Could you check a few things on this model? Use its own coordinates, in mm. A direction names the side the tool comes from. Round coordinates to 2 decimals unless told otherwise and drop trailing zeros. Loops run counter-clockwise (first coordinate to the right, second up) from the corner with the lowest first, then second, coordinate; pieces in that order, holes last.
from build123d import *

# Parameters (mm, degrees)
SKETCH1_W           = 109.51405142
SKETCH1_H           = 53
SKETCH1_R           = 1.75
BOSS_EXTRUDE1_DEPTH = 30
SKETCH2_W           = 93.51405142
SKETCH2_H           = 27.46
CUT_EXTRUDE1_DEPTH  = 239.893281613
SKETCH4_W           = 53.34
SKETCH4_H           = 27.94
CUT_EXTRUDE3_DEPTH  = 239.587618287
SKETCH5_W           = 56.34
SKETCH5_H           = 30.94
SKETCH5_W_2         = 53.34
SKETCH5_H_2         = 27.94
BOSS_EXTRUDE2_DEPTH = 17.78
SKETCH6_W           = 56.34
SKETCH6_H           = 30.94
BOSS_EXTRUDE3_DEPTH = 1.5
SKETCH7_W           = 7.62
SKETCH7_H           = 17.78
CUT_EXTRUDE4_DEPTH  = 237.429314807
SKETCH9_W           = 17.94
SKETCH9_H           = 2.25
CUT_EXTRUDE5_DEPTH  = 5
SKETCH10_W          = 8
SKETCH10_H          = 11.94
CUT_EXTRUDE6_DEPTH  = 2.54
SKETCH13_W          = 10
SKETCH13_H          = 37.94
CUT_EXTRUDE8_DEPTH  = 1
FILLET2_R           = 1
SKETCH11_W          = 27.660998728
SKETCH11_H          = 1.943421484
CUT_EXTRUDE7_DEPTH  = 126.308928087
SKETCH14_W          = 50.91
SKETCH14_H          = 49.656
SKETCH14_R          = 19.812
SKETCH14_R_2        = 1.7
BOSS_EXTRUDE4_DEPTH = 2.54
SKETCH15_W          = 8
SKETCH15_H          = 8
SKETCH15_R          = 1.7
SKETCH15_W_2        = 9.25
BOSS_EXTRUDE5_DEPTH = 27.94
SKETCH16_R          = 26.289
CUT_EXTRUDE9_DEPTH  = 2.54
CUT_EXTRUDE2_DEPTH  = 1.5
CUT_EXTRUDE11_DEPTH = 1


with BuildPart() as part:
    # Sketch1 → Boss-Extrude1 (new body)
    with BuildSketch(Plane(origin=(0, 0, 0), x_dir=(1, 0, 0), z_dir=(0, 1, 0))):
        with Locations((-176.24297429, 26.5)):
            Rectangle(SKETCH1_W, SKETCH1_H)
        with Locations(Location((-227.083491572, 41.4, 0), (0, 0, 270))):
            Circle(SKETCH1_R, mode=Mode.SUBTRACT)
        with Locations(Location((-227.083491572, 2.501598642, 0), (0, 0, 270))):
            Circle(SKETCH1_R, mode=Mode.SUBTRACT)
        with Locations(Location((-125.40594858, 41.4, 0), (0, 0, 270))):
            Circle(SKETCH1_R, mode=Mode.SUBTRACT)
        with Locations(Location((-125.40594858, 2.501598642, 0), (0, 0, 270))):
            Circle(SKETCH1_R, mode=Mode.SUBTRACT)
    extrude(amount=BOSS_EXTRUDE1_DEPTH)

    # Sketch2 → Cut-Extrude1 (cut, through all)
    with BuildSketch(Plane.XY):
        with Locations((-176.24297429, 16.27)):
            Rectangle(SKETCH2_W, SKETCH2_H)
    extrude(amount=-CUT_EXTRUDE1_DEPTH, mode=Mode.SUBTRACT)

    # Sketch4 → Cut-Extrude3 (cut, through all)
    with BuildSketch(Plane(origin=(0, 2.54, 0), x_dir=(1, 0, 0), z_dir=(0, 1, 0))):
        with Locations((-176.24297429, 26.5)):
            Rectangle(SKETCH4_W, SKETCH4_H)
    extrude(amount=-CUT_EXTRUDE3_DEPTH, mode=Mode.SUBTRACT)

    # Sketch5 → Boss-Extrude2 (add)
    with BuildSketch(Plane(origin=(0, 2.54, 0), x_dir=(1, 0, 0), z_dir=(0, 1, 0))):
        with Locations((-176.24297429, 26.5)):
            Rectangle(SKETCH5_W, SKETCH5_H)
        with Locations((-176.24297429, 26.5)):
            Rectangle(SKETCH5_W_2, SKETCH5_H_2, mode=Mode.SUBTRACT)
    extrude(amount=BOSS_EXTRUDE2_DEPTH)

    # Sketch6 → Boss-Extrude3 (add)
    with BuildSketch(Plane(origin=(0, 20.32, 0), x_dir=(1, 0, 0), z_dir=(0, 1, 0))):
        with Locations((-176.24297429, 26.5)):
            Rectangle(SKETCH6_W, SKETCH6_H)
    extrude(amount=BOSS_EXTRUDE3_DEPTH)

    # Sketch7 → Cut-Extrude4 (cut, through all)
    with BuildSketch(Plane.XY.offset(-40.47)):
        with Locations((-153.38297429, 11.43)):
            Rectangle(SKETCH7_W, SKETCH7_H)
    extrude(amount=-CUT_EXTRUDE4_DEPTH, mode=Mode.SUBTRACT)

    # Sketch9 → Cut-Extrude5 (cut)
    with BuildSketch(Plane(origin=(-202.91297429, 0, 0), x_dir=(0, 0, -1), z_dir=(1, 0, 0))):
        with Locations((26.5, 1.665)):
            Rectangle(SKETCH9_W, SKETCH9_H)
    extrude(amount=-CUT_EXTRUDE5_DEPTH, mode=Mode.SUBTRACT)

    # Sketch10 → Cut-Extrude6 (cut)
    with BuildSketch(Plane.XZ):
        with Locations((-145.57297429, -26.5)):
            Rectangle(SKETCH10_W, SKETCH10_H)
    extrude(amount=-CUT_EXTRUDE6_DEPTH, mode=Mode.SUBTRACT)

    # Sketch13 → Cut-Extrude8 (cut)
    with BuildSketch(Plane.XZ):
        with Locations((-154.57297429, -26.5)):
            Rectangle(SKETCH13_W, SKETCH13_H)
    extrude(amount=-CUT_EXTRUDE8_DEPTH, mode=Mode.SUBTRACT)

    # Fillet2
    # the kernel refuses this fillet: 1 mm, written as the material it takes off along each edge
    with BuildSketch(Plane(origin=(-149.07297429, 20.82, -40.97), x_dir=(0, 1, 0), z_dir=(1, 0, 0))) as fillet2_piece_1_section:
        Polygon((0, 0), (FILLET2_R * 1.02, 0), (FILLET2_R * 1.02, -FILLET2_R * 1.02), (0, -FILLET2_R * 1.02), align=None)
    fillet2_piece_1 = extrude(amount=FILLET2_R * 1.02, mode=Mode.PRIVATE)
    fillet2_piece_1 = fillet2_piece_1 - Plane(origin=(-149.07297429, 20.82, -40.97), x_dir=(0, -0.7071067811865475, 0.7071067811865475), z_dir=(1, 0, 0)) * Sphere(FILLET2_R, mode=Mode.PRIVATE)
    add(fillet2_piece_1, mode=Mode.SUBTRACT)
    with BuildSketch(Plane(origin=(-149.07297429, 20.82, -12.03), x_dir=(0, 1, 0), z_dir=(1, 0, 0))) as fillet2_piece_2_section:
        Polygon((0, 0), (FILLET2_R * 1.02, 0), (FILLET2_R * 1.02, FILLET2_R * 1.02), (0, FILLET2_R * 1.02), align=None)
    fillet2_piece_2 = extrude(amount=FILLET2_R * 1.02, mode=Mode.PRIVATE)
    fillet2_piece_2 = fillet2_piece_2 - Plane(origin=(-149.07297429, 20.82, -12.03), x_dir=(0, -0.7071067811865475, -0.7071067811865475), z_dir=(1, 0, 0)) * Sphere(FILLET2_R, mode=Mode.PRIVATE)
    add(fillet2_piece_2, mode=Mode.SUBTRACT)
    with BuildSketch(Plane(origin=(-157.19297429, 20.32, -40.47), x_dir=(0, 0, -1), z_dir=(0, -1, 0))) as fillet2_piece_3:
        with BuildLine():
            CenterArc((FILLET2_R, -FILLET2_R), FILLET2_R, 90, 90)
            Line((0, -FILLET2_R), (0, 0))
            Line((0, 0), (FILLET2_R, 0))
        make_face()
    extrude(amount=17.78, mode=Mode.SUBTRACT)
    with BuildSketch(Plane(origin=(-148.07297429, 2.54, -20.53), x_dir=(-1, 0, 0), z_dir=(0, 0, -1)), Plane(origin=(-149.57297429, 2.54, -20.53), x_dir=(0, 1, 0), z_dir=(0, 0, -1))) as fillet2_piece_4:
        with BuildLine():
            CenterArc((FILLET2_R, FILLET2_R), FILLET2_R, 180, 90)
            Line((0, FILLET2_R), (0, 0))
            Line((0, 0), (FILLET2_R, 0))
        make_face()
    extrude(amount=11.94, mode=Mode.SUBTRACT)
    with BuildSketch(Plane(origin=(-207.91297429, 2.54, -17.53), x_dir=(-1, 0, 0), z_dir=(0, 0, -1))) as fillet2_piece_5:
        with BuildLine():
            CenterArc((FILLET2_R, -FILLET2_R), FILLET2_R, 90, 90)
            Line((0, -FILLET2_R), (0, 0))
            Line((0, 0), (FILLET2_R, 0))
        make_face()
    extrude(amount=17.94, mode=Mode.SUBTRACT)
    with BuildSketch(Plane(origin=(-204.41297429, 2.79, -35.47), x_dir=(1, 0, 0), z_dir=(0, 0, 1))) as fillet2_piece_6:
        with BuildLine():
            CenterArc((FILLET2_R, FILLET2_R), FILLET2_R, 180, 90)
            Line((0, FILLET2_R), (0, 0))
            Line((0, 0), (FILLET2_R, 0))
        make_face()
    extrude(amount=17.94, mode=Mode.SUBTRACT)
    with BuildSketch(Plane(origin=(-157.19297429, 20.32, -41.97), x_dir=(0, 0, 1), z_dir=(0, -1, 0))) as fillet2_piece_7:
        with BuildLine():
            CenterArc((FILLET2_R, FILLET2_R), FILLET2_R, 180, 90)
            Line((0, FILLET2_R), (0, 0))
            Line((0, 0), (FILLET2_R, 0))
        make_face()
    extrude(amount=17.78, mode=Mode.SUBTRACT)
    with BuildSketch(Plane(origin=(-206.91297429, 21.82, -41.97), x_dir=(0, 0, 1), z_dir=(1, 0, 0)), Plane(origin=(-149.07297429, 21.82, -11.03), x_dir=(0, 0, -1), z_dir=(-1, 0, 0))) as fillet2_piece_8:
        with BuildLine():
            CenterArc((FILLET2_R, FILLET2_R), FILLET2_R, 180, 90)
            Line((0, FILLET2_R), (0, 0))
            Line((0, 0), (FILLET2_R, 0))
        make_face()
    extrude(amount=57.84, mode=Mode.SUBTRACT)
    with BuildSketch(Plane(origin=(-204.41297429, 2.54, -41.97), x_dir=(0, 0, 1), z_dir=(0, 1, 0))) as fillet2_piece_9:
        with BuildLine():
            CenterArc((FILLET2_R, FILLET2_R), FILLET2_R, 180, 90)
            Line((0, FILLET2_R), (0, 0))
            Line((0, 0), (FILLET2_R, 0))
        make_face()
    extrude(amount=21.78, mode=Mode.SUBTRACT)
    with BuildSketch(Plane(origin=(-148.07297429, 2.54, -41.97), x_dir=(0, 0, 1), z_dir=(0, 1, 0))) as fillet2_piece_10:
        with BuildLine():
            CenterArc((FILLET2_R, -FILLET2_R), FILLET2_R, 90, 90)
            Line((0, -FILLET2_R), (0, 0))
            Line((0, 0), (FILLET2_R, 0))
        make_face()
    extrude(amount=18.28, mode=Mode.SUBTRACT)
    with BuildSketch(Plane(origin=(-148.07297429, 21.82, -40.97), x_dir=(0, -1, 0), z_dir=(0, 0, 1))) as fillet2_piece_11:
        with BuildLine():
            CenterArc((FILLET2_R, -FILLET2_R), FILLET2_R, 90, 90)
            Line((0, -FILLET2_R), (0, 0))
            Line((0, 0), (FILLET2_R, 0))
        make_face()
    extrude(amount=28.94, mode=Mode.SUBTRACT)
    with BuildSketch(Plane(origin=(-148.07297429, 2.54, -11.03), x_dir=(0, 0, -1), z_dir=(0, 1, 0))) as fillet2_piece_12:
        with BuildLine():
            CenterArc((FILLET2_R, FILLET2_R), FILLET2_R, 180, 90)
            Line((0, FILLET2_R), (0, 0))
            Line((0, 0), (FILLET2_R, 0))
        make_face()
    extrude(amount=18.28, mode=Mode.SUBTRACT)
    with BuildSketch(Plane(origin=(-204.41297429, 24.32, -11.03), x_dir=(1, 0, 0), z_dir=(0, -1, 0))) as fillet2_piece_13:
        with BuildLine():
            CenterArc((FILLET2_R, -FILLET2_R), FILLET2_R, 90, 90)
            Line((0, -FILLET2_R), (0, 0))
            Line((0, 0), (FILLET2_R, 0))
        make_face()
    extrude(amount=21.78, mode=Mode.SUBTRACT)

    # Sketch11 → Cut-Extrude7 (cut, through all)
    with BuildSketch(Plane.ZY.offset(231)):
        with Locations((-22.072453187, 29.028289258)):
            Rectangle(SKETCH11_W, SKETCH11_H)
    extrude(amount=-CUT_EXTRUDE7_DEPTH, mode=Mode.SUBTRACT)

    # Sketch14 → Boss-Extrude4 (add)
    with BuildSketch(Plane.XZ):
        with Locations((-256.455, -24.828)):
            Rectangle(SKETCH14_W, SKETCH14_H)
        with Locations(Location((-257.078, -24.828, 0), (0, 0, 270))):
            Circle(SKETCH14_R, mode=Mode.SUBTRACT)
        with Locations(Location((-277.906, -45.656, 0), (0, 0, 270))):
            Circle(SKETCH14_R_2, mode=Mode.SUBTRACT)
        with Locations(Location((-236.25, -45.656, 0), (0, 0, 270))):
            Circle(SKETCH14_R_2, mode=Mode.SUBTRACT)
        with Locations(Location((-236.25, -4, 0), (0, 0, 270))):
            Circle(SKETCH14_R_2, mode=Mode.SUBTRACT)
        with Locations(Location((-277.906, -4, 0), (0, 0, 270))):
            Circle(SKETCH14_R_2, mode=Mode.SUBTRACT)
    extrude(amount=-BOSS_EXTRUDE4_DEPTH)

    # Sketch15 → Boss-Extrude5 (add)
    # profile 1 of 4: a face of its own
    with BuildSketch(Plane(origin=(0, 2.54, 0), x_dir=(1, 0, 0), z_dir=(0, 1, 0))):
        with Locations((-277.91, 45.656)):
            Rectangle(SKETCH15_W, SKETCH15_H)
        with Locations(Location((-277.906, 45.656, 0), (0, 0, 90))):
            Circle(SKETCH15_R, mode=Mode.SUBTRACT)
    # profile 2 of 4: a face of its own
    with BuildSketch(Plane(origin=(0, 2.54, 0), x_dir=(1, 0, 0), z_dir=(0, 1, 0))):
        with Locations((-235.625, 45.656)):
            Rectangle(SKETCH15_W_2, SKETCH15_H)
        with Locations(Location((-236.25, 45.656, 0), (0, 0, 90))):
            Circle(SKETCH15_R, mode=Mode.SUBTRACT)
    # profile 3 of 4: a face of its own
    with BuildSketch(Plane(origin=(0, 2.54, 0), x_dir=(1, 0, 0), z_dir=(0, 1, 0))):
        with Locations((-235.625, 4)):
            Rectangle(SKETCH15_W_2, SKETCH15_H)
        with Locations(Location((-236.25, 4, 0), (0, 0, 90))):
            Circle(SKETCH15_R, mode=Mode.SUBTRACT)
    # profile 4 of 4: a face of its own
    with BuildSketch(Plane(origin=(0, 2.54, 0), x_dir=(1, 0, 0), z_dir=(0, 1, 0))):
        with Locations((-277.91, 4)):
            Rectangle(SKETCH15_W, SKETCH15_H)
        with Locations(Location((-277.906, 4, 0), (0, 0, 90))):
            Circle(SKETCH15_R, mode=Mode.SUBTRACT)
    extrude(amount=BOSS_EXTRUDE5_DEPTH)

    # Sketch16 → Cut-Extrude9 (cut)
    with BuildSketch(Plane(origin=(0, 30.48, 0), x_dir=(1, 0, 0), z_dir=(0, 1, 0))):
        with Locations((-257.078, 24.828)):
            Circle(SKETCH16_R)
    extrude(amount=-CUT_EXTRUDE9_DEPTH, mode=Mode.SUBTRACT)

    # Sketch3 → Cut-Extrude2 (cut, symmetric)
    with BuildSketch(Plane(origin=(0, 20, 0), x_dir=(1, 0, 0), z_dir=(0, 1, 0))):
        Polygon((-123.673897772, 5.501598642), (-121.48594858, 5.501598642), (-121.48594858, -0.498401358), (-123.673897772, -0.498401358), (-127.137999388, -0.498401358), (-128.870050195, 2.501598642), (-127.137999388, 5.501598642), align=None)
        Polygon((-121.48594858, 44.4), (-123.673897772, 44.4), (-127.137999388, 44.4), (-128.870050195, 41.4), (-127.137999388, 38.4), (-123.673897772, 38.4), (-121.48594858, 38.4), align=None)
        Polygon((-228.812050808, 5.501598642), (-230.545843893, 2.504616343), (-228.817281138, -0.495377574), (-225.347949192, -0.498401358), (-222.995024046, -0.498401358), (-222.995024046, 5.501598642), align=None)
        Polygon((-228.812050808, 44.4), (-230.545843893, 41.403017701), (-228.817281138, 38.403023784), (-225.347949192, 38.4), (-223, 38.4), (-223, 44.4), align=None)
    extrude(amount=CUT_EXTRUDE2_DEPTH, both=True, mode=Mode.SUBTRACT)

    # Sketch17 → Cut-Extrude11 (cut)
    with BuildSketch(Plane.XZ):
        with BuildLine():
            Line((-141.57297429, -20.53), (-141.57297429, -32.47))
            ThreePointArc((-141.57297429, -32.47), (-135.60297429, -26.5), (-141.57297429, -20.53))
        make_face()
    extrude(amount=-CUT_EXTRUDE11_DEPTH, mode=Mode.SUBTRACT)


solid = part.part
Item 1: For faces 5 (the flat face through (-229.67, 20.02, -42.92)), 6 (the flat face through (-240.25, 16, -46)), 7 (the flat face through (-275, 27.94, -7)), 8 (the flat face through (-123, 18.5, -3)), which set-ups out of +Z, -Z, +X, -X, +Y, -Y let a thin tool reach every point of the face, with its end or its side?
Results list:
face 5: none
face 6: +Z, -Z, +Y
face 7: +Y
face 8: +X
Item 2: If we section it at B-B, the plane z = -15: Please give me the cut outline in (x, y), then the cut area to 3 significant figures.
Results list:
outline: (-281.91, 0) - (-274.28, 0) - (-274.28, 2.54) - (-281.91, 2.54) - close; (-239.88, 0) - (-202.91, 0) - (-202.91, 20.32) - (-149.57, 20.32) - (-149.57, 0) - (-121.49, 0) - (-121.49, 28.06) - (-129.49, 28.06) - (-129.49, 2.54) - (-148.07, 2.54) - (-148.07, 20.82) arc R1 ccw to (-149.07, 21.82) - (-204.41, 21.82) - (-204.41, 2.54) - (-223, 2.54) - (-223, 28.06) - (-231, 28.06) - (-231, 2.54) - (-239.88, 2.54) - close
area: 731 mm2
Item 3: If we section it at D-D, the plane x = -211: Please give me the cut outline in (y, z), then the cut area to 3 significant figures.
Results list:
outline: (0, -53) - (2.54, -53) - (2.54, 0) - (0, 0) - close
area: 135 mm2
Item 4: If I drill on line 1 along Z through (x, y) = (-236, 1); line 2 along X through (y, z) = (6.5, -27.5); line 3 along X through (y, z) = (23, -22), over which ranges is the centre line in solid material (lowest first)?
Results list:
line 1: z = -49.66 to -47.34, -43.97 to -5.68, -2.32 to 0
line 2: x = -231 to -223, -204.41 to -202.91, -149.57 to -148.07, -129.49 to -121.49
line 3: x = -231 to -223, -129.49 to -121.49
Item 5: We'd pull the mould along Y, two halves only. Please class faces 1 (the flat face through (-227, 30, -5)), 2 (the flat face through (-124, 20, -5.502)), 3 (the cylindrical face through (-275.645, 29.228, -43.439)), 4 (the flat face through (-205, 1, -35.47)): released by +Y, released by -Y, zero draft, split by the parting line, or undercut.
Results list:
face 1: released by +Y
face 2: undercut
face 3: zero draft
face 4: undercut
Item 6: If we section it at C-C, the plane y = 10: Count the separate pieces of the cut face and the enclosed holes in it, then the cut area to 3 significant figures.
Results list:
separate pieces: 5
enclosed holes: 8
area: 1,290 mm2
Item 7: Will these pins go through, and if not, where does the flat tip stop? pin 1 (5.5 mm diameter, centred on x = -206, z = -25, fed in from +Y); pin 2 (2.5 mm diameter, centred on x = -123.5, z = -5.5, fed in from +Y); pin 3 (2 mm diameter, centred on y = 26, z = -40.5, fed in from -X).
Results list:
pin 1: stops at y = 21.82
pin 2: stops at y = 30
pin 3: stops at x = -231
Item 8: If we section it at A-A, the plane x = -152: Please give me the cut outline in (y, z), then the cut area to 3 significant figures.
Results list:
outline: (0, -53) - (2.54, -53) - (2.54, -40.47) - (1, -40.47) - (1, -45.47) - (0, -45.47) - close; (0, -7.53) - (1, -7.53) - (1, -12.53) - (20.32, -12.53) - (20.32, -41.97) - (20.82, -41.97) arc R1 ccw to (21.82, -40.97) - (21.82, -12.03) arc R1 ccw to (20.82, -11.03) - (2.54, -11.03) - (2.54, 0) - (0, 0) - close
area: 126 mm2
